Part model, mm, in its own coordinate system. Face numbers are marked on the shaded views. A direction names the side the tool comes from. Give positions to 0.01 mm unless a question says otherwise; leave off trailing zeros. Loops run counter-clockwise (first coordinate to the right, second up) from the corner with the lowest first, then second, coordinate; pieces in that order, holes last. Notation, with made-up numbers: M 65,-39 L 97,-39 A24 cw 97,-27 Z; hole C 78.5,58 d7. An arc over 180 degrees is marked long. Put each result on its own line as item: value. Start each with the question number.
Autodesk Inventor part; units mm, degrees
ref_plane "YZ Plane" through (0, 0, 0) normal (1, 0, 0) x (0, 1, 0)
ref_plane "XZ Plane" through (0, 0, 0) normal (0, 1, 0) x (-1, 0, 0)
ref_plane "XY Plane" through (0, 0, 0) normal (0, 0, 1) x (1, 0, 0)
sketch "Sketch1" plane through (0, 0, 0) normal (0, 0, 1) x (1, 0, 0)
  line L0 (-22.5, -22.5) -> (22.5, -22.5)
  line L1 (22.5, -22.5) -> (22.5, 22.5)
  line L2 (22.5, 22.5) -> (-22.5, 22.5)
  line L3 (-22.5, 22.5) -> (-22.5, -22.5)
  line L4 (-22.5, -22.5) -> (22.5, 22.5) construction
  line L5 (22.5, -22.5) -> (-22.5, 22.5) construction
  line L6 (-17.5, -17.5) -> (17.5, -17.5)
  line L7 (17.5, -17.5) -> (17.5, 17.5)
  line L8 (17.5, 17.5) -> (-17.5, 17.5)
  line L9 (-17.5, 17.5) -> (-17.5, -17.5)
  line L10 (-17.5, -17.5) -> (17.5, 17.5) construction
  line L11 (17.5, -17.5) -> (-17.5, 17.5) construction
  line L12 (-22.5, 17.5) -> (22.5, 17.5)
  point P0 (0, 0)
  dimension "d0" = 45
  dimension "d20" = 5
  dimension "d21" = 5
extrude "Extrusion1" add sketch "Sketch1" along normal blind 60 contours L3 L12 L9 L6 L7 L1 L0 | L3 L2 L1 L12 L8
sketch "Sketch2" plane through (0, 0, 0) normal (0, 0, -1) x (-1, 0, 0)
  line L0 (17.5, -17.5) -> (17.5, 17.5)
  line L1 (-17.5, -17.5) -> (17.5, -17.5)
  line L2 (17.5, -17.5) -> (17.5, 17.5)
  line L3 (17.5, 17.5) -> (-17.5, 17.5)
  line L4 (-17.5, 17.5) -> (-17.5, -17.5)
  line L5 (-17.5, -17.5) -> (17.5, 17.5) construction
  line L6 (17.5, -17.5) -> (-17.5, 17.5) construction
  line L7 (-22.5, 22.5) -> (22.5, 22.5)
  line L8 (-22.5, -22.5) -> (22.5, -22.5)
  line L9 (22.5, -22.5) -> (22.5, 22.5)
  line L10 (22.5, 22.5) -> (-22.5, 22.5)
  line L11 (-22.5, 22.5) -> (-22.5, -22.5)
  line L12 (-22.5, -22.5) -> (22.5, 22.5) construction
  line L13 (22.5, -22.5) -> (-22.5, 22.5) construction
  line L14 (-39.1057, 22.5) -> (57.4203, 22.5)
  point P0 (0, 0)
  dimension "d18" = 5
  dimension "d19" = 5
revolve "Revolution1" add sketch "Sketch2" angle 90 about axis through (39.1057, 22.5, 0) along (1, 0, 0)
sketch "Sketch3" plane through (-22.5, 22.5, 60) normal (0, 1, 0) x (1, 0, 0)
  line L0 (5, 65) -> (5, 100)
  line L1 (40, 85) -> (5, 85)
  line L2 (5, 85) -> (5, 100)
  line L3 (5, 100) -> (40, 100)
  line L4 (35.2339, 98.1928) -> (5, 100) construction
  line L5 (5, 85) -> (35.2339, 113.1928) construction
  line L6 (0, 60) -> (0, 105)
  line L7 (45, 80) -> (0, 80)
  line L8 (0, 80) -> (0, 105)
  line L9 (0, 105) -> (45, 105)
  line L10 (40.2339, 93.1928) -> (0, 105) construction
  line L11 (0, 80) -> (45, 122.7171) construction
  line L12 (40, 100) -> (40, 65)
  line L13 (40, 100) -> (40, 85)
  line L14 (45, 105) -> (45, 0)
  line L15 (45, 105) -> (45, 80)
  point P0 (22.5, 60)
  point P1 (20.117, 99.0964)
  point P2 (43.816, 121.1954)
  point P3 (20.117, 99.0964)
  point P4 (0, 80)
  point P5 (5, 85)
  dimension "d17" = 15
extrude "Extrusion2" add sketch "Sketch3" along normal blind 50
extrude "Extrusion4" add sketch "Sketch1" against normal blind 25 contours L3 L2 L1 L12 L8
extrude "Extrusion5" cut sketch "Sketch3" along normal blind 75.5 contours L0 L3 L12 L1
sketch "Sketch10" plane through (-22.5, 72.5, 60) normal (0, 1, 0) x (1, 0, 0)
  line L0 (45, 105) -> (0, 105)
  line L1 (0, 105) -> (0, 80)
  line L2 (0, 80) -> (45, 80)
  line L3 (45, 80) -> (45, 105)
  line L4 (5, 100) -> (40, 100)
  line L5 (40, 85) -> (5, 85)
  line L6 (40, 100) -> (5, 100)
  line L7 (5, 100) -> (5, 85)
  line L8 (5, 85) -> (40, 85)
  line L9 (40, 85) -> (40, 100)
  line L10 (-3.6161, 80) -> (47.5585, 80)
revolve "Revolution3" add sketch "Sketch10" angle 90 about axis through (-26.1161, 72.5, -20) along (1, 0, 0)
sketch "Sketch11" plane through (-22.5, 22.5, -20) normal (0, 0, 1) x (1, 0, 0)
  line L0 (45, 75) -> (0, 75)
  line L1 (45, 50) -> (0, 50)
  line L2 (45, 75) -> (0, 75)
  line L3 (0, 75) -> (0, 50)
  line L4 (0, 50) -> (45, 50)
  line L5 (45, 50) -> (45, 75)
  line L6 (40, 70) -> (40, 55)
  line L7 (40, 55) -> (5, 55)
  line L8 (40, 70) -> (5, 70)
  line L9 (5, 70) -> (5, 55)
  line L10 (5, 55) -> (40, 55)
  line L11 (40, 55) -> (40, 70)
  point P0 (22.5, -22.5)
  dimension "d68" = 15
extrude "Extrusion8" add sketch "Sketch11" along normal blind 80
sketch "Sketch12" plane through (-22.5, 22.5, 60) normal (0, 1, 0) x (1, 0, 0)
  point P0 (22.5, 60)
sketch "Sketch13" plane through (0, 0, 60) normal (0, 0, 1) x (1, 0, 0)
  line L0 (17.5, 17.5) -> (17.5, -17.5)
  line L1 (17.5, 17.5) -> (19.8638, 17.5)
  line L2 (19.8638, 17.5) -> (19.8638, 20.41)
  line L3 (19.8638, 20.41) -> (17.5, 20.41)
  line L4 (17.5, 20.41) -> (17.5, 17.5)
  line L5 (17.5, -17.5) -> (19.8638, -17.5)
  line L6 (19.8638, -17.5) -> (19.8638, -20.6538)
  line L7 (19.8638, -20.6538) -> (17.5, -20.6538)
  line L8 (17.5, -20.6538) -> (17.5, -17.5)
  point P0 (0, 0)
extrude "Extrusion9" cut sketch "Sketch13" against normal blind 80.25
sketch "Sketch14" plane through (-22.5, 22.5, 60) normal (0, 1, 0) x (1, 0, 0)
  circle A0 centre (33.1575, 35) radius 4
  line L0 (45, 0) -> (0, 0)
  point P0 (22.5, 60)
  dimension "d72" = 8
  dimension "d73" = 35
extrude "Extrusion10" cut sketch "Sketch14" against normal blind 28.5
properties material "Iron, Malleable"
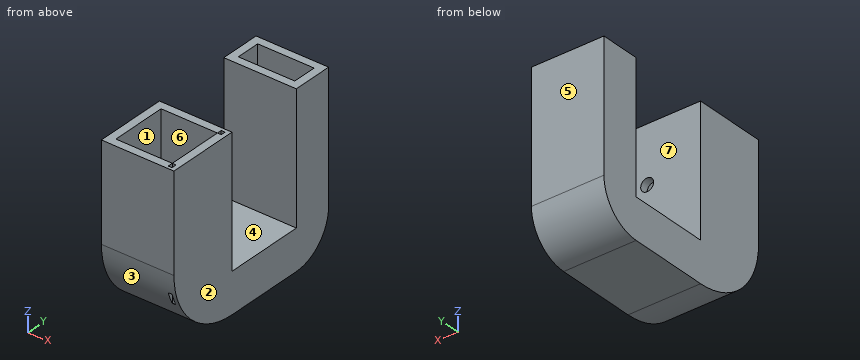
1) Band-saw the part on D-D on y = 62.5. Give the cut face in (x, z).
2) Mould opens along Z. For the marked faces 1, 2, 3 and 4 say: +Z half, -Z half, draft (parallel to the pull), parting line (faces both ways), or undercut.
3) Band-saw the part on C-C on x = -2. Give the cut face in (y, z), then the cut area to 3 significant figures.
4) Wall check: L1, parallel to Y at x = 4, z = 11; L2, parallel to X at y = 19, z = 25; L3, parallel to Y at x = 18.5, z = 37. Give the ranges that are in metal, low to high.
5) Pin check, flat tips, straight feed: pin 1 Ø10.5 at (x, y) = (8.5, 36) entering from +Z; pin 2 Ø5 at (x, y) = (-10.5, 4) entering from +Z; pin 3 Ø1.2 at (x, y) = (18.5, 19) entering from +Z; pin 4 Ø12 at (x, y) = (-6.5, 18) entering from -Z. Stop position of each tip, or through.
6) Which spindle directions (+Z, -Z, +X, -X, +Y, -Y) get a long thin tool onto all of the face, cutting with end or side? Do the marked faces 5, 6 and 7. Say none if no direction does.
Evaluation:
1. outline: M -22.5,-45 L 22.5,-45 L 22.5,-20 L -22.5,-20 Z; hole M -17.5,-40 L 17.5,-40 L 17.5,-25 L -17.5,-25 Z
2. face 1: undercut
2. face 2: draft
2. face 3: -Z half
2. face 4: +Z half
3. outline: M -22.5,0 A45 ccw 22.5,-45 L 72.5,-45 A25 ccw 97.5,-20 L 97.5,60 L 92.5,60 L 92.5,-20 A20 cw 72.5,-40 L 22.5,-40 A40 cw -17.5,0 L -17.5,60 L -22.5,60 Z; M 17.5,-25 L 72.5,-25 A5 ccw 77.5,-20 L 77.5,60 L 72.5,60 L 72.5,-20 L 22.5,-20 L 22.5,60 L 17.5,60 Z
3. area: 2,560 mm2
4. L1: -22.5 to -17.5, 17.5 to 22.5, 72.5 to 77.5, 92.5 to 97.5
4. L2: -22.5 to 6.66, 14.66 to 17.5, 19.86 to 22.5
4. L3: -22.5 to -20.65, -17.5 to 17.5, 20.41 to 22.5, 72.5 to 97.5
5. pin 1: z = -20
5. pin 2: z = -34.04
5. pin 3: z = -20.25
5. pin 4: z = -45
6. face 5: +Z, -Z, +X, -X, +Y
6. face 6: +Z
6. face 7: +Z, +X, -X
